Design review of the part built by this model. Coordinates are the model's own, in mm. A direction names the side the tool comes from. Coordinates: 2 decimals unless noted, no trailing zeros. Write each loop counter-clockwise with the first axis right and the second up, starting at its lowest first coordinate (ties: lowest second). Pieces come first, ordered by that corner, then holes. Notation, with made-up numbers: (31.5, 34.5) - (70.5, 34.5) arc R22 ccw to (70.5, 69.5) - close; hole circle Ø11 at (75.25, -28). An arc over 180 degrees is marked (long way). Answer as CSV lines item,"result". Start each with the question number.
Q1. Machinability: for faces 1 (the face through (1, 50, -35)), 2 (the face through (-1, 65, 20)), 3 (the face through (-124.99, 49.58, -0.77)), which of the approach directions +Z, -Z, +X, -X, +Y, -Y give a long, thin tool a straight path to every point of the face, cutting with its end or side? Answer none if there is none.
Q2. We need section A-A (z = 0). Write out the cut boundary in (x, y), plus the area to 4 significant figures.
Q3. Mouldability with a two-part tool opening along X and no side actions: class faces 4 (the face through (110, 65, 0)), 5 (the face through (34, 20, -51)), 6 (the face through (164.98, 9.86, 1.65)) as pulls with the +X half, pulls with the -X half, needs draft (parallel to the pull), parting line crosses it, or undercut.
Q4. We need section B-B (y = 57). Write out the cut boundary in (x, z).
Q5. For line 1 along X through (y, z) = (14, -55); line 2 along Z through (x, y) = (15, 66); line 3 along Y through (x, z) = (120.5, -44), list the stretches that pass through material, from the lowest coordinate up. Write a range as [from, to].
Q6. Clearance check with flat-ended pins moving along their axes: pin 1 (8 mm diameter, centred on x = 70, y = 54.5, fed in from +Z); pin 2 (12 mm diameter, centred on x = 54, y = 52.5, fed in from -Z); pin 3 (20 mm diameter, centred on x = -51.5, z = 6, fed in from +Y). State where each tip first meets the part, or that it passes through.
Q7. We need section D-D (y = 27.5). Write out the cut boundary in (x, z).
Q8. We need section C-C (x = 0). Write out the cut boundary in (y, z).
from build123d import *

# Parameters (mm, degrees)
SKETCH1_R           = 10
SKETCH1_R_2         = 7.5
BOSS_EXTRUDE1_DEPTH = 20
SKETCH1_4_R         = 7.5
BOSS_EXTRUDE2_DEPTH = 50
BOSS_EXTRUDE3_DEPTH = 80


with BuildPart() as part:
    # Sketch1 → Boss-Extrude1 (new body)
    # profile 1 of 3: a face of its own
    with BuildSketch(Plane(origin=(0, 0, 0), x_dir=(1, 0, 0), z_dir=(0, 1, 0))):
        with BuildLine():
            Line((90, 75), (-90, 75))
            ThreePointArc((-90, 75), (-165, 0), (-90, -75))
            Line((-90, -75), (90, -75))
            ThreePointArc((90, -75), (165, 0), (90, 75))
        make_face()
        with Locations(Location((90, -55, 0), (0, 0, 270))):
            Circle(SKETCH1_R, mode=Mode.SUBTRACT)
        with Locations(Location((90, 55, 0), (0, 0, 270))):
            Circle(SKETCH1_R, mode=Mode.SUBTRACT)
        with Locations(Location((0, -55, 0), (0, 0, 270))):
            Circle(SKETCH1_R, mode=Mode.SUBTRACT)
        with Locations(Location((0, 55, 0), (0, 0, 270))):
            Circle(SKETCH1_R, mode=Mode.SUBTRACT)
        with Locations(Location((-90, -55, 0), (0, 0, 270))):
            Circle(SKETCH1_R, mode=Mode.SUBTRACT)
        with Locations(Location((-90, 55, 0), (0, 0, 270))):
            Circle(SKETCH1_R, mode=Mode.SUBTRACT)
        with BuildLine():
            ThreePointArc((-90, 35), (-125, 0), (-90, -35))
            Line((-90, -35), (90, -35))
            ThreePointArc((90, -35), (125, 0), (90, 35))
            Line((90, 35), (-90, 35))
        make_face(mode=Mode.SUBTRACT)
    # profile 2 of 3: a face of its own
    with BuildSketch(Plane(origin=(0, 0, 0), x_dir=(1, 0, 0), z_dir=(0, 1, 0))):
        with BuildLine():
            Line((90, 35), (-90, 35))
            ThreePointArc((-90, 35), (-125, 0), (-90, -35))
            Line((-90, -35), (90, -35))
            ThreePointArc((90, -35), (125, 0), (90, 35))
        make_face()
        with BuildLine():
            ThreePointArc((-90, 20), (-110, 0), (-90, -20))
            Line((-90, -20), (90, -20))
            ThreePointArc((90, -20), (110, 0), (90, 20))
            Line((90, 20), (-90, 20))
        make_face(mode=Mode.SUBTRACT)
    # profile 3 of 3: a face of its own
    with BuildSketch(Plane(origin=(0, 0, 0), x_dir=(1, 0, 0), z_dir=(0, 1, 0))):
        with BuildLine():
            Line((90, 20), (-90, 20))
            ThreePointArc((-90, 20), (-110, 0), (-90, -20))
            Line((-90, -20), (90, -20))
            ThreePointArc((90, -20), (110, 0), (90, 20))
        make_face()
        with Locations(Location((-90, 0, 0), (0, 0, 270))):
            Circle(SKETCH1_R_2, mode=Mode.SUBTRACT)
        with Locations(Location((0, 0, 0), (0, 0, 270))):
            Circle(SKETCH1_R_2, mode=Mode.SUBTRACT)
        with Locations(Location((90, 0, 0), (0, 0, 270))):
            Circle(SKETCH1_R_2, mode=Mode.SUBTRACT)
    extrude(amount=BOSS_EXTRUDE1_DEPTH)

    # Sketch1_4 → Boss-Extrude2 (add)
    with BuildSketch(Plane(origin=(0, 0, 0), x_dir=(1, 0, 0), z_dir=(0, 1, 0))):
        with BuildLine():
            Line((90, 20), (-90, 20))
            ThreePointArc((-90, 20), (-110, 0), (-90, -20))
            Line((-90, -20), (90, -20))
            ThreePointArc((90, -20), (110, 0), (90, 20))
        make_face()
        with Locations(Location((-90, 0, 0), (0, 0, 270))):
            Circle(SKETCH1_4_R, mode=Mode.SUBTRACT)
        with Locations(Location((0, 0, 0), (0, 0, 270))):
            Circle(SKETCH1_4_R, mode=Mode.SUBTRACT)
        with Locations(Location((90, 0, 0), (0, 0, 270))):
            Circle(SKETCH1_4_R, mode=Mode.SUBTRACT)
    extrude(amount=BOSS_EXTRUDE2_DEPTH)

    # Sketch1_5 → Boss-Extrude3 (add)
    with BuildSketch(Plane(origin=(0, 0, 0), x_dir=(1, 0, 0), z_dir=(0, 1, 0))):
        with BuildLine():
            Line((90, 35), (-90, 35))
            ThreePointArc((-90, 35), (-125, 0), (-90, -35))
            Line((-90, -35), (90, -35))
            ThreePointArc((90, -35), (125, 0), (90, 35))
        make_face()
        with BuildLine():
            ThreePointArc((-90, 20), (-110, 0), (-90, -20))
            Line((-90, -20), (90, -20))
            ThreePointArc((90, -20), (110, 0), (90, 20))
            Line((90, 20), (-90, 20))
        make_face(mode=Mode.SUBTRACT)
    extrude(amount=BOSS_EXTRUDE3_DEPTH)


solid = part.part
Results list:
1,face 1,"-Z, +X, -X, +Y"
1,face 2,"+Y"
1,face 3,"-X, +Y"
2,outline,"(-165, 0) - (-97.5, 0) - (-97.5, 50) - (-110, 50) - (-110, 80) - (-125, 80) - (-125, 20) - (-165, 20) - close; (-82.5, 0) - (-7.5, 0) - (-7.5, 50) - (-82.5, 50) - close; (7.5, 0) - (82.5, 0) - (82.5, 50) - (7.5, 50) - close; (97.5, 0) - (165, 0) - (165, 20) - (125, 20) - (125, 80) - (110, 80) - (110, 50) - (97.5, 50) - close"
2,area,"12,750 mm2"
3,face 4,"undercut"
3,face 5,"needs draft"
3,face 6,"pulls with the +X half"
4,outline,"(-90, -35) - (90, -35) arc R35 ccw to (90, 35) - (-90, 35) arc R35 ccw to start; hole (-90, -20) - (90, -20) arc R20 ccw to (90, 20) - (-90, 20) arc R20 ccw to start"
5,line 1,"x = [-140.99, -100], [-80, -10], [10, 80], [100, 140.99]"
5,line 2,"z = [-35, -20], [20, 35]"
5,line 3,"y = [0, 20]"
6,pin 1,"stops at z = 35"
6,pin 2,"stops at z = -35"
6,pin 3,"stops at y = 50"
7,outline,"(-90, -35) - (90, -35) arc R35 ccw to (90, 35) - (-90, 35) arc R35 ccw to start; hole circle Ø15 at (-90, 0); hole circle Ø15 at (0, 0); hole circle Ø15 at (90, 0)"
8,outline,"(0, -75) - (20, -75) - (20, -65) - (0, -65) - close; (0, -45) - (20, -45) - (20, -35) - (80, -35) - (80, -20) - (50, -20) - (50, -7.5) - (0, -7.5) - close; (0, 7.5) - (50, 7.5) - (50, 20) - (80, 20) - (80, 35) - (20, 35) - (20, 45) - (0, 45) - close; (0, 65) - (20, 65) - (20, 75) - (0, 75) - close"
